Geometry check sheet. Reference: the model listing, model coordinates, mm. A direction names the side the tool comes from. Round coordinates to 2 decimals unless told otherwise and drop trailing zeros. Loops run counter-clockwise (first coordinate to the right, second up) from the corner with the lowest first, then second, coordinate; pieces in that order, holes last. Notation, with made-up numbers: (14, 15.5) - (38, 15.5) arc R19 cw to (38, 45.5) - close; hole circle Ø11 at (64, 9). An arc over 180 degrees is marked (long way). Write item = value, one per line.
```python
from build123d import *

# Parameters (mm, degrees)
SKETCH_1_W               = 25
SKETCH_1_H               = 25
EXTRUDE_1_DEPTH          = 3
SKETCH_2_W               = 3
SKETCH_2_H               = 100
EXTRUDE_2_DEPTH          = 190
FILLET_1_R               = 10
SKETCH_3_W               = 20
SKETCH_3_H               = 15
CUT_EXTRUDE_2_DEPTH      = 10
FILLET_2_R               = 10
FILLET_3_R               = 10
CUT_EXTRUDE_3_DEPTH      = 5
CUT_EXTRUDE_3_DEPTH_BACK = 5
SKETCH_4_R               = 1.05
SKETCH_4_R_2             = 1


with BuildPart() as part:
    # 草图1 → 凸台-拉伸1 (new body)
    with BuildSketch(Plane.XY):
        with Locations((-100.141216583, -61.148491789)):
            Rectangle(SKETCH_1_W, SKETCH_1_H)
    extrude(amount=EXTRUDE_1_DEPTH)

    # 草图2 → 凸台-拉伸2 (add)
    with BuildSketch(Plane.XY.offset(3)):
        with Locations((-89.141216583, -23.452816851)):
            Rectangle(SKETCH_2_W, SKETCH_2_H)
    extrude(amount=EXTRUDE_2_DEPTH)

    # 圆角1
    fillet_1_edges = [part.edges().sort_by_distance(p)[0] for p in [
        (-90.641216583, -61.05065432, 3),
    ]]
    fillet(fillet_1_edges, radius=FILLET_1_R)

    # 草图3 → 切除-拉伸2 (cut)
    with BuildSketch(Plane(origin=(-87.641216583, 0, 0), x_dir=(0, 0, -1), z_dir=(1, 0, 0))):
        with Locations((-25, 4.047183149)):
            Rectangle(SKETCH_3_W, SKETCH_3_H)
        with Locations((-55, 4.047183149)):
            Rectangle(SKETCH_3_W, SKETCH_3_H)
        with Locations((-85, 4.047183149)):
            Rectangle(SKETCH_3_W, SKETCH_3_H)
        with Locations((-115, 4.047183149)):
            Rectangle(SKETCH_3_W, SKETCH_3_H)
        with Locations((-145, 4.047183149)):
            Rectangle(SKETCH_3_W, SKETCH_3_H)
        with Locations((-175, 4.047183149)):
            Rectangle(SKETCH_3_W, SKETCH_3_H)
        with Locations((-55, -22.952816851)):
            Rectangle(SKETCH_3_W, SKETCH_3_H)
        with Locations((-85, -22.952816851)):
            Rectangle(SKETCH_3_W, SKETCH_3_H)
        with Locations((-115, -22.952816851)):
            Rectangle(SKETCH_3_W, SKETCH_3_H)
        with Locations((-145, -22.952816851)):
            Rectangle(SKETCH_3_W, SKETCH_3_H)
        with Locations((-175, -22.952816851)):
            Rectangle(SKETCH_3_W, SKETCH_3_H)
        with Locations((-55, -49.952816851)):
            Rectangle(SKETCH_3_W, SKETCH_3_H)
        with Locations((-85, -49.952816851)):
            Rectangle(SKETCH_3_W, SKETCH_3_H)
        with Locations((-115, -49.952816851)):
            Rectangle(SKETCH_3_W, SKETCH_3_H)
        with Locations((-145, -49.952816851)):
            Rectangle(SKETCH_3_W, SKETCH_3_H)
        with Locations((-175, -49.952816851)):
            Rectangle(SKETCH_3_W, SKETCH_3_H)
        with Locations((-25, -22.952816851)):
            Rectangle(SKETCH_3_W, SKETCH_3_H)
        with Locations((-25, -49.952816851)):
            Rectangle(SKETCH_3_W, SKETCH_3_H)
    extrude(amount=-CUT_EXTRUDE_2_DEPTH, mode=Mode.SUBTRACT)

    # 圆角2
    fillet_2_edges = [part.edges().sort_by_distance(p)[0] for p in [
        (-89.141216583, 26.547183149, 193),
    ]]
    fillet(fillet_2_edges, radius=FILLET_2_R)

    # 圆角3
    fillet_3_edges = [part.edges().sort_by_distance(p)[0] for p in [
        (-89.141216583, 26.547183149, 3),
    ]]
    fillet(fillet_3_edges, radius=FILLET_3_R)

    # 草图4 → 切除-拉伸3 (cut, two sides: drawn at the far end of the back side and taken through both)
    with BuildSketch(Plane.XY.offset(3).offset(-CUT_EXTRUDE_3_DEPTH_BACK)):
        with Locations((-110.141216583, -51.148491789)):
            Circle(SKETCH_4_R)
        with Locations((-110.141216583, -61.148491789)):
            Circle(SKETCH_4_R_2)
        with Locations((-110.141216583, -71.148491789)):
            Circle(SKETCH_4_R_2)
        with Locations(Location((-100.141216583, -71.148491789, 0), (0, 0, 239.999999998))):
            Circle(SKETCH_4_R_2)
        with Locations(Location((-100.141216583, -68.648491789, 0), (0, 0, 239.999999998))):
            Circle(SKETCH_4_R_2)
        with Locations(Location((-100.141216583, -51.148491789, 0), (0, 0, 239.999999998))):
            Circle(SKETCH_4_R_2)
        with Locations(Location((-100.141216583, -53.648491789, 0), (0, 0, 239.999999998))):
            Circle(SKETCH_4_R_2)
    extrude(amount=CUT_EXTRUDE_3_DEPTH + CUT_EXTRUDE_3_DEPTH_BACK, mode=Mode.SUBTRACT)


solid = part.part
```
(1) Scan lines: L1, parallel to Y at x = -90.5, z = 56.5; L2, parallel to X at y = -52.5, z = 125.5; L3, parallel to Z at x = -94.5, y = -62. Record each from-to range of solid material in increasing order. Write a range as [from, to].
Answers follow:
L1 = [-73.45, -57.45], [-42.45, -30.45], [-15.45, -3.45], [11.55, 26.55]
L2 = [-90.64, -87.64]
L3 = [0, 5.11]
(2) Section check B-B (y = -45.5). Enter the section's corners in (x, z), then the cut area to 3 significant figures.
Answers follow:
outline = (-90.64, 3) - (-87.64, 3) - (-87.64, 15) - (-90.64, 15) - close; (-90.64, 35) - (-87.64, 35) - (-87.64, 45) - (-90.64, 45) - close; (-90.64, 65) - (-87.64, 65) - (-87.64, 75) - (-90.64, 75) - close; (-90.64, 95) - (-87.64, 95) - (-87.64, 105) - (-90.64, 105) - close; (-90.64, 125) - (-87.64, 125) - (-87.64, 135) - (-90.64, 135) - close; (-90.64, 155) - (-87.64, 155) - (-87.64, 165) - (-90.64, 165) - close; (-90.64, 185) - (-87.64, 185) - (-87.64, 193) - (-90.64, 193) - close
area = 210 mm²
(3) Gauge pin test, flat ends, axial feed: pin 1 (1.5 mm diameter, centred on x = -89.5, z = 174.5, fed in from -Y); pin 2 (12 mm diameter, centred on y = -39, z = 87.5, fed in from -X); pin 3 (0.9 mm diameter, centred on x = -90, y = -22, fed in from -Z). Record the tip position at first contact, or that the pin passes through.
Answers follow:
pin_1 = -73.45
pin_2 = -90.64
pin_3 = 3
(4) Section check A-A (z = 115.5). Enter the section's corners in (x, y), then the cut area to 3 significant figures.
Answers follow:
outline = (-90.64, -73.45) - (-87.64, -73.45) - (-87.64, -57.45) - (-90.64, -57.45) - close; (-90.64, -42.45) - (-87.64, -42.45) - (-87.64, -30.45) - (-90.64, -30.45) - close; (-90.64, -15.45) - (-87.64, -15.45) - (-87.64, -3.45) - (-90.64, -3.45) - close; (-90.64, 11.55) - (-87.64, 11.55) - (-87.64, 26.55) - (-90.64, 26.55) - close
area = 165 mm²
(5) Section check C-C (x = -105.75). Enter the section's corners in (y, z), then the cut area to 3 significant figures.
Answers follow:
outline = (-73.65, 0) - (-48.65, 0) - (-48.65, 3) - (-73.65, 3) - close
area = 75.0 mm²
(6) Section check D-D (y = 14). Enter the section's corners in (x, z), then the cut area to 3 significant figures.
Answers follow:
outline = (-90.64, 3) - (-87.64, 3) - (-87.64, 193) - (-90.64, 193) - close
area = 570 mm²
(7) Set-up check for faces 1 (the flat face through (-100, -61, 0)), 2 (the flat face through (-89, -73.453, 91)), 3 (the flat face through (-90.641, -24, 97)): record each of +Z, -Z, +X, -X, +Y, -Y from which the full face is reachable in a straight line by a thin tool's end or side.
Answers follow:
face_1 = -Z, +X, -X, +Y, -Y
face_2 = +Z, +X, -X, -Y
face_3 = +Z, -X, +Y
